Verification items for this drawing (mm, ordinates from the low corner). A direction names the side the tool comes from. Round coordinates to 2 decimals unless told otherwise and drop trailing zeros. Loops run counter-clockwise (first coordinate to the right, second up) from the corner with the lowest first, then second, coordinate; pieces in that order, holes last. Notation, with made-up numbers: (29, -39.5) -> (56, -39.5) arc R14 ccw to (56, -34.5) -> close; hole circle Ø9 at (59.5, 59.5). An arc over 180 degrees is marked (long way). Use a Markdown table: item, result. Add a question column.
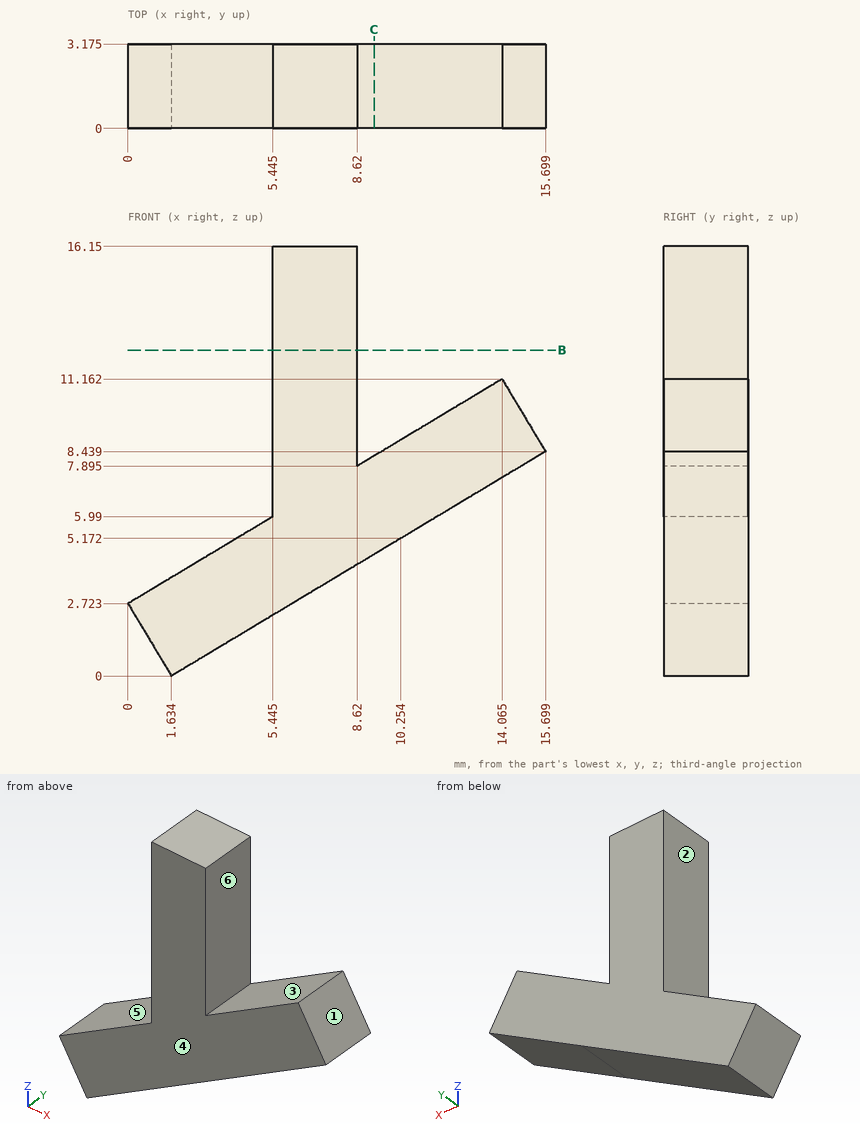
1) Access from +Z, -Z, +X, -X, +Y, -Y to the whole of each face (thin tool, end or side, straight path). Record for the marked faces 1 and 2.
2) Sectioned sample at B-B on z = 12.25. Enter the section's corners in (x, y) (1 decimal), then the cut area to 3 significant figures.
3) Sectioned sample at C-C on x = 9.25. Enter the section's corners in (y, z) (1 decimal).
4) Thickness scan on line 1 (X direction, y = 1.3, z = 14.5) (1 decimal); line 2 (X direction, y = 2.55, z = 8) (1 decimal); line 3 (X direction, y = 2.3, z = 10.5) (1 decimal). Record the ranges inside material, lowest first.
5) Go/stop test with flat-tipped pins: pin 1 (1.6 mm diameter, centred on y = 1, z = 13.5, fed in from -X) (1 decimal); pin 2 (1 mm diameter, centred on x = 3, z = 7.5, fed in from -Y); pin 3 (1.5 mm diameter, centred on y = 3, z = 4.5, fed in from +X) (1 decimal); pin 4 (1 mm diameter, centred on x = 13.5, y = 2.5, fed in from +Z). Record where each tip stops, or that it passes through.
6) Release check for a two-part mould opening along X. For the marked faces 3, 4, 5 and 6 record: released by +X, released by -X, zero draft, split by the parting line, or undercut.
Geometry results:
| question | item | result |
|---|---|---|
| 1 | face 1 | +Z, +X, +Y, -Y |
| 1 | face 2 | +Z, -X, +Y, -Y |
| 2 | outline | (5.4, 0) -> (8.6, 0) -> (8.6, 3.2) -> (5.4, 3.2) -> close |
| 2 | area | 10.1 mm^2 |
| 3 | outline | (0, 4.6) -> (3.2, 4.6) -> (3.2, 8.3) -> (0, 8.3) -> close |
| 4 | line 1 | 5.4 to 8.6 |
| 4 | line 2 | 5.4 to 8.6, 8.8 to 15 |
| 4 | line 3 | 5.4 to 8.6, 13 to 14.5 |
| 5 | pin 1 | x = 5.4 |
| 5 | pin 2 | through |
| 5 | pin 3 | x = 10.4 |
| 5 | pin 4 | z = 11.12 |
| 6 | face 3 | undercut |
| 6 | face 4 | zero draft |
| 6 | face 5 | released by -X |
| 6 | face 6 | undercut |
